```python
from build123d import *

# Parameters (mm, degrees)
F0_R     = 36.475604
F1_DEPTH = 3.7
F2_DEPTH = 8.1
F3_R     = 38.237687
F4_DEPTH = 2


with BuildPart() as f1:
    # F0 (on Top) → F1 (new body)
    with BuildSketch(Plane.XY):
        Circle(F0_R)
        Polygon((-24.211187, 17.412838), (0, 31.543903), (23.792868, 17.620649), (23.792868, -10.018051), (16.727336, -14.382056), (16.727336, -23.525685), (0, -33.292744), (-17.145654, -23.525685), (-17.145654, -14.382056), (-24.211187, -9.602431), align=None, mode=Mode.SUBTRACT)
    extrude(amount=F1_DEPTH)

    # F0 (on Top) → F2 (join)
    with BuildSketch(Plane.XY):
        Polygon((23.792868, 17.620649), (0, 31.543903), (-24.211187, 17.412838), (-24.211187, -9.602431), (-17.145654, -14.382056), (-17.145654, -23.525685), (0, -33.292744), (16.727336, -23.525685), (16.727336, -14.382056), (23.792868, -10.018051), align=None)
        Polygon((-12.534934, -21.175375), (-12.534934, -16.483145), (0, -23.52149), (11.818774, -16.734514), (11.818774, -21.175375), (0, -28.480387), align=None, mode=Mode.SUBTRACT)
        Polygon((-17.145654, 15.75036), (-17.145654, 7.23016), (-12.534934, 9.482956), (-12.534934, 18.887546), (0, 25.7752), (11.818774, 18.887546), (11.818774, 9.559093), (16.63455, 6.752592), (16.63455, 16.240098), (18.989254, 14.867842), (18.989254, -7.305608), (16.63455, -8.603099), (16.63455, -6.900904), (11.949172, -9.37198), (11.949172, -11.510435), (-0.347363, -18.396766), (-12.534934, -11.294187), (-12.534934, -9.37198), (-17.276361, -6.608808), (-17.276361, -8.542829), (-19.703554, -6.900904), (-19.703554, 14.25742), align=None, mode=Mode.SUBTRACT)
        Polygon((16.63455, 3.291251), (11.040321, 6.391475), (5.835399, 3.476604), (5.835399, -2.741615), (11.032363, -5.659703), (16.63455, -2.522355), align=None)
        Polygon((-6.036222, 3.375041), (-11.41535, 6.391475), (-17.145654, 3.182378), (-17.145654, -2.741615), (-11.562531, -6.518433), (-6.036222, -3.423579), align=None)
        Polygon((3.750607, -9.602431), (-0.347363, -2.741615), (-4.070303, -9.37198), (-0.347363, -11.890439), align=None)
    extrude(amount=F2_DEPTH)

    # F3 (on Top) → F4 (join)
    with BuildSketch(Plane.XY):
        Circle(F3_R)
    extrude(amount=-F4_DEPTH)


solid = f1.part
```
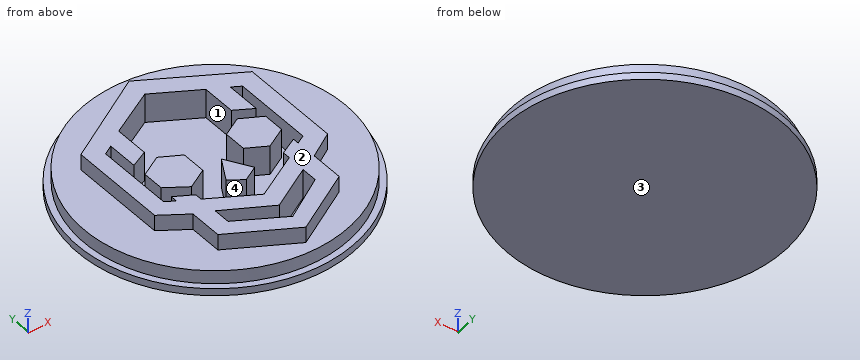
Here's how the part is built. I have some questions about the finished solid (model axes, mm). Face numbers are marked on the shaded views. A direction names the side the tool comes from. Coordinates: 2 decimals unless noted, no trailing zeros. Write each loop counter-clockwise with the first axis right and the second up, starting at its lowest first coordinate (ties: lowest second). Pieces come first, ordered by that corner, then holes. Notation, with made-up numbers: (-3, 23.5) - (45, 23.5) arc R16 ccw to (45, 28.5) - close; hole circle Ø3 at (44.5, 72.5). An arc over 180 degrees is marked (long way). One line per item, written item: value.
1) Suppose I cut it at C-C on x = -7.5. Write out the boundary of the cut face in (y, z).
Model answer:
outline: (-37.49, -2) - (37.49, -2) - (37.49, 0) - (35.7, 0) - (35.7, 3.7) - (27.17, 3.7) - (27.17, 8.1) - (21.65, 8.1) - (21.65, 0) - (4.2, 0) - (4.2, 8.1) - (-4.24, 8.1) - (-4.24, 0) - (-14.23, 0) - (-14.23, 8.1) - (-19.31, 8.1) - (-19.31, 0) - (-24.11, 0) - (-24.11, 8.1) - (-29.02, 8.1) - (-29.02, 3.7) - (-35.7, 3.7) - (-35.7, 0) - (-37.49, 0) - close
2) Suppose I cut it at B-B on y = 0. Write out the boundary of the cut face in (x, z).
Model answer:
outline: (-38.24, -2) - (38.24, -2) - (38.24, 0) - (36.48, 0) - (36.48, 3.7) - (23.79, 3.7) - (23.79, 8.1) - (18.99, 8.1) - (18.99, 0) - (16.63, 0) - (16.63, 8.1) - (5.84, 8.1) - (5.84, 0) - (-6.04, 0) - (-6.04, 8.1) - (-17.15, 8.1) - (-17.15, 0) - (-19.7, 0) - (-19.7, 8.1) - (-24.21, 8.1) - (-24.21, 3.7) - (-36.48, 3.7) - (-36.48, 0) - (-38.24, 0) - close
3) On a 3-axis mill with a long thin cutter (end or side, diameter ignored), from which of +Z, -Z, +X, -X, +Y, -Y can I reach the whole of each face in a straight line? I mean the marked faces 1 and 2. Say none if no direction works.
Model answer:
face 1: +Z
face 2: +Z, +X, -X, +Y, -Y
4) I'm going to push flat-ended pins straight in: P1, Ø2.5, axis at y = -18, z = 2.5, coming from the +X side; P2, Ø2, axis at y = -25, z = 1.5, coming from the +X side; P3, Ø3.5, axis at y = -18, z = 4, coming from the -X side. Where does each tip first touch, or does it pass through?
Model answer:
P1: stops at x = 32.4
P2: stops at x = 27.47
P3: stops at x = -32.64
5) Suppose I cut it at A-A on z = 2.5. State how many separate pieces and enclosed holes the cut face has, and give its area (3 significant figures).
Model answer:
separate pieces: 4
enclosed holes: 2
area: 3,130 mm²
6) I need wall thicknesses on line 1 along Y through (x, z) = (10.5, 0.5); line 2 along Y through (x, z) = (3, 7); line 3 along X through (y, z) = (-11, 3). Which ranges of each line are inside material? Lowest first, please.
Model answer:
line 1: y = -34.93 to -21.99, -17.49 to -12.32, -5.36 to 6.09, 19.66 to 34.93
line 2: y = -31.54 to -26.63, -21.8 to -16.52, -10.02 to -8.35, 24.03 to 29.79
line 3: x = -34.78 to -12.53, -1.66 to 1.25, 11.95 to 34.78
7) We'd pull the mould along Y, two halves only. Please class the marked faces 3 and 4: pulls with the +Y half, pulls with the -Y half, needs draft (parallel to the pull), parting line crosses it, or undercut.
Model answer:
face 3: needs draft
face 4: undercut
